Geometry: final body of the model. Coordinates: model frame, mm. A direction names the side the tool comes from. Coordinates: 2 decimals unless noted, no trailing zeros. Order: outer loops, then holes, each group sorted by start corner. A loop starts at its lowest first (then second) coordinate and runs counter-clockwise, first axis right, second up. Notation, with made-up numbers: (31, 31) -> (48, 31) arc R30 cw to (48, 69) -> close; hole circle Ø10 at (74.5, 63.5). An arc over 180 degrees is marked (long way). Use one line per item in the form item = value.
```python
from build123d import *

# Parameters (mm, degrees)
F1_DEPTH = 2
F2_DEPTH = 7


# Not quite as in the source:
# - a feature names something its author has since deleted; it is built from what else it names


with BuildPart() as f1:
    # F0 (on Top) → F1 (new body)
    with BuildSketch(Plane.XY):
        with BuildLine():
            Line((2.9579698818, 2.75), (9.6144422615, 2.75))
            ThreePointArc((9.6144422615, 2.75), (7.6537044043, 6.4359000064), (4.3588989435, 9))
            Line((4.3588989435, 9), (-1.1528000428, 9))
            Line((-1.1528000428, 9), (-1.1528000428, 2.75))
            Line((-1.1528000428, 2.75), (0, 2.75))
            Line((0, 2.75), (2.9579698818, 2.75))
        make_face()
        with BuildLine():
            ThreePointArc((-2.4256512704, -9.7013512417), (1.7468006996, -9.8462524503), (5.6147791623, -8.2749172176))
            Line((5.6147791623, -8.2749172176), (8.3706286555, -3.5016458774))
            Line((8.3706286555, -3.5016458774), (2.9579698818, -0.3766458774))
            Line((2.9579698818, -0.3766458774), (2.3815698685, -1.3749999859))
            Line((2.3815698685, -1.3749999859), (0.9025849195, -3.9366770613))
            Line((0.9025849195, -3.9366770613), (-2.4256512704, -9.7013512417))
        make_face()
        with BuildLine():
            Line((2.9579698818, -0.3766458774), (2.9579698818, 2.75))
            Line((2.9579698818, 2.75), (0, 2.75))
            ThreePointArc((0, 2.75), (1.9445436483, 1.9445436483), (2.75, 0))
            ThreePointArc((2.75, 0), (2.6562960244, -0.7117523662), (2.3815698685, -1.3749999859))
            Line((2.3815698685, -1.3749999859), (2.9579698818, -0.3766458774))
        make_face()
        with BuildLine():
            Line((-3.8605548013, 1.1866770613), (-7.1887909912, 6.9513512417))
            ThreePointArc((-7.1887909912, 6.9513512417), (-9.4005051039, 3.410352444), (-9.9736781058, -0.7250827824))
            Line((-9.9736781058, -0.7250827824), (-7.2178286127, -5.4983541226))
            Line((-7.2178286127, -5.4983541226), (-1.805169839, -2.3733541226))
            Line((-1.805169839, -2.3733541226), (-2.3815698389, -1.3750000373))
            Line((-2.3815698389, -1.3750000373), (-3.8605548013, 1.1866770613))
        make_face()
        with BuildLine():
            ThreePointArc((-2.3815698389, -1.3750000373), (-2.3815698712, 1.3749999814), (0, 2.75))
            Line((0, 2.75), (-1.1528000428, 2.75))
            Line((-1.1528000428, 2.75), (-3.8605548013, 1.1866770613))
            Line((-3.8605548013, 1.1866770613), (-2.3815698389, -1.3750000373))
        make_face()
        with BuildLine():
            Line((-1.805169839, -2.3733541226), (0.9025849195, -3.9366770613))
            Line((0.9025849195, -3.9366770613), (2.3815698685, -1.3749999859))
            ThreePointArc((2.3815698685, -1.3749999859), (2.97e-08, -2.75), (-2.3815698389, -1.3750000373))
            Line((-2.3815698389, -1.3750000373), (-1.805169839, -2.3733541226))
        make_face()
    extrude(amount=F1_DEPTH)

    # F0 (on Top) → F2 (join)
    with BuildSketch(Plane.XY):
        with BuildLine():
            Line((-1.1528000428, 9), (4.3588989435, 9))
            ThreePointArc((4.3588989435, 9), (-1.7468006996, 9.8462524503), (-7.1887909912, 6.9513512417))
            Line((-7.1887909912, 6.9513512417), (-3.8605548013, 1.1866770613))
            Line((-3.8605548013, 1.1866770613), (-1.1528000428, 2.75))
            Line((-1.1528000428, 2.75), (-1.1528000428, 9))
        make_face()
        with BuildLine():
            ThreePointArc((5.6147791623, -8.2749172176), (8.8359434025, -4.6825318139), (10, 0))
            ThreePointArc((10, 0), (9.9031414868, 1.3884483038), (9.6144422615, 2.75))
            Line((9.6144422615, 2.75), (2.9579698818, 2.75))
            Line((2.9579698818, 2.75), (2.9579698818, -0.3766458774))
            Line((2.9579698818, -0.3766458774), (8.3706286555, -3.5016458774))
            Line((8.3706286555, -3.5016458774), (5.6147791623, -8.2749172176))
        make_face()
        with BuildLine():
            ThreePointArc((-9.9736781058, -0.7250827824), (-7.6537044043, -6.4359000064), (-2.4256512704, -9.7013512417))
            Line((-2.4256512704, -9.7013512417), (0.9025849195, -3.9366770613))
            Line((0.9025849195, -3.9366770613), (-1.805169839, -2.3733541226))
            Line((-1.805169839, -2.3733541226), (-7.2178286127, -5.4983541226))
            Line((-7.2178286127, -5.4983541226), (-9.9736781058, -0.7250827824))
        make_face()
    extrude(amount=F2_DEPTH)


solid = f1.part
```
1) Section A-A, the plane z = 3.25. Output: boundary loops of the cut face in (x, y).
Results found:
outline = (-9.97, -0.73) arc R10 ccw to (-2.43, -9.7) -> (0.9, -3.94) -> (-1.81, -2.37) -> (-7.22, -5.5) -> close; (-7.19, 6.95) -> (-3.86, 1.19) -> (-1.15, 2.75) -> (-1.15, 9) -> (4.36, 9) arc R10 ccw to start; (2.96, -0.38) -> (8.37, -3.5) -> (5.61, -8.27) arc R10 ccw to (9.61, 2.75) -> (2.96, 2.75) -> close
2) Material intervals for probe 1 along Y at (x, z) = (-4.5, 4.75); probe 2 along Y at (x, z) = (0, 6.25); probe 3 along X at (y, z) = (-2.5, 2.75), sorted ascending. Write a range as from..to.
Results found:
probe_1 = -8.93..-3.93, 2.29..8.93
probe_2 = -5.5..-3.42, 9..10
probe_3 = -9.68..-8.95, -2.02..-1.59, 6.64..9.68
3) Contact query for flat-ended pins moving along their axis: P1, Ø1, axis at x = 5.5, y = 4, coming from the -Z side; P2, Ø1.5, axis at y = 7.5, z = 5, coming from the +X side; P3, Ø3.5, axis at y = 2, z = 5, coming from the -X side; P4, Ø1.5, axis at y = -8, z = 1, coming from the -X side. Output: stop coordinate, or through.
Results found:
P1 = 0
P2 = -1.15
P3 = -5.34
P4 = -6.89
4) Access query for faces 1 (the flat face through (-5.55, 4.11, 4.46)), 2 (the flat face through (-0.432, -3.166, 4.465)), 3 (the flat face through (-0.785, -6.859, 4.465)), 4 (the flat face through (-1.153, 6, 4)). Directions: +Z, -Z, +X, -X, +Y, -Y. A direction counts if a zero-diameter tool reaches every point of the face in a straight line with its end or side. Return the directions, or none.
Results found:
face_1 = +Z, -X
face_2 = +Z
face_3 = +Z, -Y
face_4 = +Z, +X
5) Section D-D, the plane x = 1.75. Output: boundary loops of the cut face in (y, z).
Results found:
outline = (-9.85, 0) -> (-2.12, 0) -> (-2.12, 2) -> (-9.85, 2) -> close; (2.12, 0) -> (9.85, 0) -> (9.85, 7) -> (9, 7) -> (9, 2) -> (2.12, 2) -> close
6) Section C-C, the plane y = -1.75. Output: boundary loops of the cut face in (x, z).
Results found:
outline = (-9.85, 0) -> (-2.12, 0) -> (-2.12, 2) -> (-9.38, 2) -> (-9.38, 7) -> (-9.85, 7) -> close; (2.12, 0) -> (9.85, 0) -> (9.85, 7) -> (5.34, 7) -> (5.34, 2) -> (2.12, 2) -> close
7) Section B-B, the plane z = 1. Output: boundary loops of the cut face in (x, y) (3 decimals), and give its area (3 significant figures).
Results found:
outline = circle Ø20 at (0, 0); hole circle Ø5.5 at (0, 0)
area = 290 mm2
8) Pull-direction query (X, two-part tool) for faces 5 (the flat face through (5.6, -1.9, 4.5)), 6 (the cylindrical face through (6.876, -7.261, 3.451)), 7 (the flat face through (2, 9, 4)); classes: released by +X, released by -X, zero draft, split by the parting line, or undercut.
Results found:
face_5 = undercut
face_6 = split by the parting line
face_7 = zero draft
